Part model, mm, in its own coordinate system. A direction names the side the tool comes from. Round coordinates to 2 decimals unless told otherwise and drop trailing zeros. Loops run counter-clockwise (first coordinate to the right, second up) from the corner with the lowest first, then second, coordinate; pieces in that order, holes last. Notation, with made-up numbers: M -12,-25 L 28,-25 A13 ccw 28,0 Z; hole C 32.25,65 d10. An arc over 180 degrees is marked long. Answer as CSV lines item,"result". Start each with the question number.
Item 1: Which spindle directions (+Z, -Z, +X, -X, +Y, -Y) get a long thin tool onto all of the face, cutting with end or side? Do faces 4 (the flat face through (10.55, 6, 4)), 5 (the flat face through (9, -3.55, 4)), 6 (the flat face through (-15, 0, 1)), 7 (the flat face through (9, -7.55, 4)), 8 (the flat face through (-2.55, -4, 2)). Say none if no direction does.
Item 2: Band-saw the part on A-A (z = 0.35). Give the cut face in (x, y).
Item 3: Mould opens along Y. For faces 1 (the flat face through (9, 7.55, 4)), 2 (the flat face through (2, -4.55, 2)), 3 (the flat face through (-4, 3, 0)) say: pulls with the +Y half, pulls with the -Y half, needs draft (parallel to the pull), parting line crosses it, or undercut.
Item 4: Wall check: line 1 (Y direction, x = -3, z = 1.3); line 2 (X direction, y = -1, z = 0.4); line 3 (Y direction, x = -12, z = 0.6). Give the ranges that are in metal, low to high.
Item 5: Band-saw the part on B-B (x = -7). Give the cut face in (y, z), and give its area (3 significant figures).
Item 6: Band-saw the part on C-C (y = 0.55). Give the cut face in (x, z).
Item 7: Band-saw the part on D-D (z = 4.65). Give the cut face in (x, y), and give its area (3 significant figures).
Item 8: Drop flat-ended pins along their axis: pin 1 Ø0.6 at (y, z) = (-6.5, 4.5) entering from -X; pin 2 Ø2.5 at (x, y) = (-12.85, 0.55) entering from +Z; pin 3 Ø3.5 at (x, y) = (-12, -9.5) entering from +Z; pin 4 Ø1 at (y, z) = (-5.5, 4) entering from +X. Give the stop position or say it passes through.
```python
from build123d import *

# Parameters (mm, degrees)
SKETCH_1_W          = 30
SKETCH_1_H          = 25
EXTRUDE_1_DEPTH     = 3
CUT_EXTRUDE_1_DEPTH = 20.754746265
SKETCH_3_W          = 4
SKETCH_3_H          = 4
SKETCH_3_W_2        = 3
EXTRUDE_2_DEPTH     = 2
FILLET_1_R          = 3
SKETCH_4_R          = 1.5
CUT_EXTRUDE_2_DEPTH = 21.155644371
SKETCH_5_R          = 1.5
CUT_EXTRUDE_3_DEPTH = 8


with BuildPart() as part:
    # 草图1 → 凸台-拉伸1 (new body)
    with BuildSketch(Plane.XY):
        Rectangle(SKETCH_1_W, SKETCH_1_H)
    extrude(amount=EXTRUDE_1_DEPTH)

    # 草图2 → 切除-拉伸1 (cut, through all)
    with BuildSketch(Plane.XY.offset(3)):
        Polygon((6.55, 0), (6.55, 4.55), (-2.55, 4.55), (-2.55, 2.7), (-8.45, 2.7), (-8.45, 0), (-8.45, -2.7), (-2.55, -2.7), (-2.55, -4.55), (6.55, -4.55), align=None)
    extrude(amount=-CUT_EXTRUDE_1_DEPTH, mode=Mode.SUBTRACT)

    # 草图3 → 凸台-拉伸2 (add)
    with BuildSketch(Plane.XY.offset(3)):
        with Locations((8.55, 5.55)):
            Rectangle(SKETCH_3_W, SKETCH_3_H)
        with Locations((9.05, -5.55)):
            Rectangle(SKETCH_3_W_2, SKETCH_3_H)
    extrude(amount=EXTRUDE_2_DEPTH)

    # 圆角1
    fillet_1_edges = [part.edges().sort_by_distance(p)[0] for p in [
        (-15, 12.5, 1.5),
        (15, 12.5, 1.5),
        (15, -12.5, 1.5),
        (-15, -12.5, 1.5),
    ]]
    fillet(fillet_1_edges, radius=FILLET_1_R)

    # 草图4 → 切除-拉伸2 (cut, through all)
    with BuildSketch(Plane(origin=(0, 0, 0), x_dir=(-1, 0, 0), z_dir=(0, 0, -1))):
        with Locations((12, -9.5)):
            Circle(SKETCH_4_R)
        with Locations((-12, -9.5)):
            Circle(SKETCH_4_R)
    extrude(amount=-CUT_EXTRUDE_2_DEPTH, mode=Mode.SUBTRACT)

    # 草图5 → 切除-拉伸3 (cut)
    with BuildSketch(Plane(origin=(0, 0, 0), x_dir=(-1, 0, 0), z_dir=(0, 0, -1))):
        with Locations((12.85, 0.55)):
            Circle(SKETCH_5_R)
    extrude(amount=-CUT_EXTRUDE_3_DEPTH, mode=Mode.SUBTRACT)


solid = part.part
```
Answer block:
1,face 4,"+Z, +X, +Y, -Y"
1,face 5,"+Z, +X, -X"
1,face 6,"+Z, -Z, -X, +Y, -Y"
1,face 7,"+Z, +X, -X, -Y"
1,face 8,"+Z, -Z"
2,outline,"M -15,-9.5 A3 ccw -12,-12.5 L 12,-12.5 A3 ccw 15,-9.5 L 15,9.5 A3 ccw 12,12.5 L -12,12.5 A3 ccw -15,9.5 Z; hole C -12.85,0.55 d3; hole C -12,-9.5 d3; hole M -8.45,-2.7 L -2.55,-2.7 L -2.55,-4.55 L 6.55,-4.55 L 6.55,4.55 L -2.55,4.55 L -2.55,2.7 L -8.45,2.7 Z; hole C 12,-9.5 d3"
3,face 1,"pulls with the +Y half"
3,face 2,"undercut"
3,face 3,"needs draft"
4,line 1,"y = -12.5 to -2.7, 2.7 to 12.5"
4,line 2,"x = -15 to -8.45, 6.55 to 15"
4,line 3,"y = -12.5 to -11, -8 to -0.69, 1.79 to 12.5"
5,outline,"M -12.5,0 L -2.7,0 L -2.7,3 L -12.5,3 Z; M 2.7,0 L 12.5,0 L 12.5,3 L 2.7,3 Z"
5,area,"58.8 mm^2"
6,outline,"M -15,0 L -14.35,0 L -14.35,3 L -15,3 Z; M -11.35,0 L -8.45,0 L -8.45,3 L -11.35,3 Z; M 6.55,0 L 15,0 L 15,3 L 6.55,3 Z"
7,outline,"M 6.55,3.55 L 10.55,3.55 L 10.55,7.55 L 6.55,7.55 Z; M 7.55,-7.55 L 10.55,-7.55 L 10.55,-3.55 L 7.55,-3.55 Z"
7,area,"28.0 mm^2"
8,pin 1,"stops at x = 7.55"
8,pin 2,"passes through"
8,pin 3,"stops at z = 3"
8,pin 4,"stops at x = 10.55"
